```python
from build123d import *

# Parameters (mm, degrees)
F0_W            = 57.15
F0_H            = 25.4
F1_DEPTH        = 11.176
F2_W            = 57.15
F2_H            = 8.3099603653
F3_DEPTH        = 32.639
F5_DEPTH        = 3.81
F6_DEPTH        = 16.8559801826
F8_DEPTH        = 3.81
F10_D           = 4.2164
F10_CBORE_D     = 7.112
F10_CBORE_DEPTH = 9.652
F11_D           = 3.4544
F11_DEPTH       = 12.03325
F11_TIP         = 1.0378064612


with BuildPart() as f1:
    # F0 (on Top) → F1 (new body)
    with BuildSketch(Plane.XY):
        Rectangle(F0_W, F0_H)
    extrude(amount=F1_DEPTH)

    # F2 (on face) → F3 (join)
    with BuildSketch(Plane.XY.offset(11.176)):
        Rectangle(F2_W, F2_H)
    extrude(amount=F3_DEPTH)

    # F4 (on face) → F5 (cut)
    with BuildSketch(Plane.XZ.offset(4.1549801826)):
        with BuildLine():
            ThreePointArc((17.526, 30.8229), (16.6407009568, 32.9602009568), (14.5034, 33.8455))
            Line((14.5034, 33.8455), (-14.5034, 33.8455))
            ThreePointArc((-14.5034, 33.8455), (-16.6407009568, 32.9602009568), (-17.526, 30.8229))
            Line((-17.526, 30.8229), (-17.526, 24.1681))
            ThreePointArc((-17.526, 24.1681), (-16.6407009568, 22.0307990432), (-14.5034, 21.1455))
            Line((-14.5034, 21.1455), (14.5034, 21.1455))
            ThreePointArc((14.5034, 21.1455), (16.6407009568, 22.0307990432), (17.526, 24.1681))
            Line((17.526, 24.1681), (17.526, 30.8229))
        make_face()
    extrude(amount=-F5_DEPTH, mode=Mode.SUBTRACT)

    # F4 (on face) → F6 (cut, through all)
    with BuildSketch(Plane.XZ.offset(4.1549801826)):
        with BuildLine():
            ThreePointArc((-17.526, 42.6742546607), (-16.6407009568, 40.5369537039), (-14.5034, 39.6516546607))
            Line((-14.5034, 39.6516546607), (14.5034, 39.6516546607))
            ThreePointArc((14.5034, 39.6516546607), (16.6407009568, 40.5369537039), (17.526, 42.6742546607))
            Line((17.526, 42.6742546607), (17.526, 43.815))
            Line((17.526, 43.815), (-17.526, 43.815))
            Line((-17.526, 43.815), (-17.526, 42.6742546607))
        make_face()
    extrude(amount=-F6_DEPTH, mode=Mode.SUBTRACT)

    # F7 (on face) → F8 (cut)
    with BuildSketch(Plane(origin=(0, 4.1549801826, 0), x_dir=(-1, 0, 0), z_dir=(0, 1, 0))):
        with BuildLine():
            ThreePointArc((-14.5034, 33.8455), (-16.6407009568, 32.9602009568), (-17.526, 30.8229))
            Line((-17.526, 30.8229), (-17.526, 24.1681))
            ThreePointArc((-17.526, 24.1681), (-16.6407009568, 22.0307990432), (-14.5034, 21.1455))
            Line((-14.5034, 21.1455), (14.5034, 21.1455))
            ThreePointArc((14.5034, 21.1455), (16.6407009568, 22.0307990432), (17.526, 24.1681))
            Line((17.526, 24.1681), (17.526, 30.8229))
            ThreePointArc((17.526, 30.8229), (16.6407009568, 32.9602009568), (14.5034, 33.8455))
            Line((14.5034, 33.8455), (-14.5034, 33.8455))
        make_face()
    extrude(amount=-F8_DEPTH, mode=Mode.SUBTRACT)

    # F10 (through all)
    with Locations(Plane(origin=(0, 0, 0), x_dir=(1, 0, 0), z_dir=(0, 0, -1))):
        with Locations((-22.987, 0), (22.987, 0)):
            CounterBoreHole(F10_D / 2, F10_CBORE_D / 2, F10_CBORE_DEPTH)

    # F11
    with Locations(Plane(origin=(0, 0, 0), x_dir=(1, 0, 0), z_dir=(0, 0, -1))):
        with Locations((-15.875, 0), (15.875, 0)):
            Hole(F11_D / 2, depth=F11_DEPTH)
            with Locations((0, 0, -(F11_DEPTH + F11_TIP / 2))):  # 118° drill point
                Cone(0, F11_D / 2, F11_TIP, mode=Mode.SUBTRACT)


solid = f1.part
```
Part model, mm, in its own coordinate system. A direction names the side the tool comes from. Give positions to 0.01 mm unless a question says otherwise; leave off trailing zeros. Write each loop counter-clockwise with the first axis right and the second up, starting at its lowest first coordinate (ties: lowest second). Pieces come first, ordered by that corner, then holes. Notation, with made-up numbers: (63, 44.5) -> (68, 44.5) arc R23 ccw to (68, 67.5) -> close; hole circle Ø6 at (82.25, 15). An arc over 180 degrees is marked (long way). Put each result on its own line as item: value. Start each with the question number.
Item 1: Pin check, flat tips, straight feed: pin 1 Ø3 at (x, y) = (22, 1) entering from -Z; pin 2 Ø9 at (x, y) = (-7, -1.5) entering from +Z; pin 3 Ø10 at (x, z) = (-6, 30.5) entering from +Y (3 decimals). Stop position of each tip, or through.
Item 2: Cut at B-B (x = 3). List the corners of the cut face in (y, z).
Item 3: Which spindle directions (+Z, -Z, +X, -X, +Y, -Y) get a long thin tool onto all of the face, cutting with end or side? Do faces 1 (the face through (-16.62, 2.28, 22.01)), 2 (the face through (16.617, -0.058, 40.514)), 3 (the face through (0, -4.155, 20)), 4 (the face through (-26.54, -0.16, 4.76)). Say none if no direction does.
Item 4: Cut at C-C (x = -24). List the corners of the cut face in (y, z) (3 decimals), then the cut area to 3 significant figures.
Item 5: Wall check: L1, parallel to Z at x = -8.5, y = 0.5; L2, parallel to Z at x = 25.5, y = -9; L3, parallel to Y at x = -22, z = 4. Give the ranges that are in metal, low to high. Write a range as [from, to].
Item 6: Cut at A-A (z = 17). List the corners of the cut face in (x, y) (3 decimals), then the cut area to 3 significant figures.
Item 7: Pull direction X, two halves, no side cores. Call faces 5 (the face through (0, 2, 21.146)), 6 (the face through (0, 4.155, 20)): pulls with the +X half, pulls with the -X half, needs draft (parallel to the pull), parting line crosses it, or undercut.
Item 8: Cut at D-D (y = 9.25). List the corners of the cut face in (x, z) (3 decimals), then the cut area to 3 significant figures.
Answer list:
1. pin 1: stops at z = 9.65
1. pin 2: stops at z = 39.65
1. pin 3: stops at y = 4.155
2. outline: (-12.7, 0) -> (12.7, 0) -> (12.7, 11.18) -> (4.15, 11.18) -> (4.15, 21.15) -> (0.34, 21.15) -> (0.34, 33.85) -> (4.15, 33.85) -> (4.15, 39.65) -> (-4.15, 39.65) -> (-4.15, 33.85) -> (-0.34, 33.85) -> (-0.34, 21.15) -> (-4.15, 21.15) -> (-4.15, 11.18) -> (-12.7, 11.18) -> close
3. face 1: +Y
3. face 2: +Z, +Y, -Y
3. face 3: +Z, +X, -X, -Y
3. face 4: -Z
4. outline: (-12.7, 0) -> (-3.409, 0) -> (-3.409, 9.652) -> (-1.849, 9.652) -> (-1.849, 43.815) -> (-4.155, 43.815) -> (-4.155, 11.176) -> (-12.7, 11.176) -> close; (1.849, 9.652) -> (3.409, 9.652) -> (3.409, 0) -> (12.7, 0) -> (12.7, 11.176) -> (4.155, 11.176) -> (4.155, 43.815) -> (1.849, 43.815) -> close
4. area: 363 mm2
5. L1: z = [0, 21.15], [33.85, 39.65]
5. L2: z = [0, 11.18]
5. L3: y = [-12.7, -3.42], [3.42, 12.7]
6. outline: (-28.575, -4.155) -> (28.575, -4.155) -> (28.575, 4.155) -> (-28.575, 4.155) -> close; hole circle Ø4.216 at (-22.987, 0); hole circle Ø4.216 at (22.987, 0)
6. area: 447 mm2
7. face 5: undercut
7. face 6: needs draft
8. outline: (-28.575, 0) -> (28.575, 0) -> (28.575, 11.176) -> (-28.575, 11.176) -> close
8. area: 639 mm2
